The listing builds one solid part. Answer for the finished solid, in the listing's coordinates (mm). A direction names the side the tool comes from. Coordinates: 2 decimals unless noted, no trailing zeros. Loops run counter-clockwise (first coordinate to the right, second up) from the corner with the lowest first, then second, coordinate; pieces in that order, holes last. Notation, with made-up numbers: M 88.5,-1.5 L 93.5,-1.5 A21 ccw 93.5,9.5 Z; hole C -14,31.25 d1. An arc over 180 degrees is marked long. Return JSON: item names as keys, results as strings. Group by question number.
1. Which of the six approach directions +Z, -Z, +X, -X, +Y, -Y give full straight-line access (tool end or side, diameter ignored) to faces 4 (the face through (-34.312, 32.734, 0.493)), 5 (the face through (-52.69, -0.96, 0.49))?
2. The mould has two halves that part along Y. Classify faces 1 (the face through (-24.191, 53.748, 0.493)), 2 (the face through (-51, 0, 1)), 3 (the face through (-46.606, 15.187, 0.493)): pulls with the +Y half, pulls with the -Y half, needs draft (parallel to the pull), parting line crosses it, or undercut.
3. Straight lines are drawn through the part: L1, parallel to Y at x = -55.5, z = 0.25; L2, parallel to Y at x = -23.5, z = 0.75; L3, parallel to X at y = -23, z = 0.5. For each, find the intervals that lie inside material, in ascending order. Write a range as from..to.
4. Section C-C (z = 0.8) is taken. Count the separate pieces of the cut face and the enclosed holes in it, then the cut area to 3 significant figures.
5. Given P1, Ø4.5, axis at x = -55, y = 0, coming from the -Z side, flat-ended and moving along its own axis, determine where the tip first touches the part or whether it passes through.
6. Section A-A (x = -55.5) is taken. Write down the section's boundary in (y, z), then the cut area to 3 significant figures.
7. Section B-B (y = 0) is taken. Write down the section's boundary in (x, z).
```python
from build123d import *

# Parameters (mm, degrees)
IZIM1_R                     = 2.5
Y_KSEKLIK_EKSTR_ZYON1_DEPTH = 1


with BuildPart() as part:
    # Çizim1 → Yükseklik-Ekstrüzyon1 (new body)
    with BuildSketch(Plane.XY):
        with BuildLine():
            Line((-23.446136356, -44.161959762), (-25.73775467, -42.866863479))
            Line((-25.73775467, -42.866863479), (-26.834295942, -39.938466016))
            ThreePointArc((-26.834295942, -39.938466016), (-28.201527977, -38.125336415), (-30.335428898, -37.348658075))
            Line((-30.335428898, -37.348658075), (-33.334907776, -37.164700371))
            Line((-33.334907776, -37.164700371), (-33.842709051, -34.202800331))
            ThreePointArc((-33.842709051, -34.202800331), (-34.84597704, -32.165592505), (-36.7965457, -31.002818113))
            Line((-36.7965457, -31.002818113), (-39.708425324, -30.260072511))
            Line((-39.708425324, -30.260072511), (-39.652227319, -27.255483394))
            ThreePointArc((-39.652227319, -27.255483394), (-40.255989993, -25.066366444), (-41.954126526, -23.558687864))
            Line((-41.954126526, -23.558687864), (-44.675252109, -22.283466496))
            Line((-44.675252109, -22.283466496), (-44.057045667, -19.342627369))
            ThreePointArc((-44.057045667, -19.342627369), (-44.239914432, -17.079151855), (-45.625461503, -15.279979352))
            Line((-45.625461503, -15.279979352), (-48.059435816, -13.517457571))
            Line((-48.059435816, -13.517457571), (-46.901121207, -10.744549126))
            ThreePointArc((-46.901121207, -10.744549126), (-46.656617846, -8.486899797), (-47.680491761, -6.459969953))
            Line((-47.680491761, -6.459969953), (-49.741090048, -4.272585973))
            Line((-49.741090048, -4.272585973), (-48.083701146, -1.765839874))
            ThreePointArc((-48.083701146, -1.765839874), (-47.420487313, 0.406004917), (-48.046416828, 2.588887101))
            Line((-48.046416828, 2.588887101), (-49.660641368, 5.123644113))
            Line((-49.660641368, 5.123644113), (-47.562892001, 7.275425136))
            ThreePointArc((-47.562892001, 7.275425136), (-46.504462376, 9.284526705), (-46.710273625, 11.546031539))
            Line((-46.710273625, 11.546031539), (-47.82093971, 14.338366552))
            Line((-47.82093971, 14.338366552), (-45.357143694, 16.058954583))
            ThreePointArc((-45.357143694, 16.058954583), (-43.940993675, 17.834139505), (-43.719395692, 20.094152054))
            Line((-43.719395692, 20.094152054), (-44.287157421, 23.045145208))
            Line((-44.287157421, 23.045145208), (-41.54459596, 24.273587558))
            ThreePointArc((-41.54459596, 24.273587558), (-39.820893366, 25.751969023), (-39.17973637, 27.930427214))
            Line((-39.17973637, 27.930427214), (-39.184480502, 30.935538106))
            Line((-39.184480502, 30.935538106), (-36.260310201, 31.628316593))
            ThreePointArc((-36.260310201, 31.628316593), (-34.290118058, 32.757522199), (-33.252115355, 34.777253066))
            Line((-33.252115355, 34.777253066), (-32.693673826, 37.730024144))
            Line((-32.693673826, 37.730024144), (-29.691484877, 37.862596744))
            ThreePointArc((-29.691484877, 37.862596744), (-27.544598222, 38.602623821), (-26.146521576, 40.39207739))
            Line((-26.146521576, 40.39207739), (-25, 43.301270189))
            ThreePointArc((-25, 43.301270189), (-24.226890609, 43.73851588), (-23.446136356, 44.161959762))
            ThreePointArc((-23.446136356, 44.161959762), (-21.212806241, 47.755648425), (-21.906244367, 51.929556087))
            ThreePointArc((-21.906244367, 51.929556087), (-24.232021318, 53.76021953), (-27.179564099, 53.490852446))
            ThreePointArc((-27.179564099, 53.490852446), (-59.999999835, 0.004450967), (-27.1875, -53.486819346))
            Line((-27.1875, -53.486819346), (-27.179564099, -53.490852446))
            ThreePointArc((-27.179564099, -53.490852446), (-24.232021318, -53.76021953), (-21.906244367, -51.929556087))
            ThreePointArc((-21.906244367, -51.929556087), (-21.212806241, -47.755648425), (-23.446136356, -44.161959762))
        make_face()
        with Locations((-31.620079453, -45.001895242)):
            Circle(IZIM1_R, mode=Mode.SUBTRACT)
        with Locations((-55, 0)):
            Circle(IZIM1_R, mode=Mode.SUBTRACT)
        with Locations((-28.000624989, 47.338831842)):
            Circle(IZIM1_R, mode=Mode.SUBTRACT)
    extrude(amount=Y_KSEKLIK_EKSTR_ZYON1_DEPTH)


solid = part.part
```
Worked out:
{
 "1": {"face 4": "+Z, -Z, +X", "face 5": "+Z, -Z"},
 "2": {"face 1": "pulls with the +Y half", "face 2": "needs draft", "face 3": "undercut"},
 "3": {"L1": "-22.8..-2.45, 2.45..22.8", "L2": "-53.46..-44.13, 44.13..53.46", "L3": "-55.42..-43.15"},
 "4": {"separate pieces": "1", "enclosed holes": "3", "area": "1,380 mm^2"},
 "5": {"P1": "through"},
 "6": {"outline": "M -22.8,0 L -2.45,0 L -2.45,1 L -22.8,1 Z; M 2.45,0 L 22.8,0 L 22.8,1 L 2.45,1 Z", "area": "40.7 mm^2"},
 "7": {"outline": "M -60,0 L -57.5,0 L -57.5,1 L -60,1 Z; M -52.5,0 L -47.44,0 L -47.44,1 L -52.5,1 Z"}
}
